from build123d import *

# Parameters (mm, degrees)
ENL_V_MAT_EXTRU_1_DEPTH      = 0.7
R_P_TITION_CIRCULAIRE1_COUNT = 4
ENL_V_MAT_EXTRU_2_REACH      = 75.418
ESQUISSE3_R                  = 1.25


with BuildPart() as part:
    # Esquisse1 → Révolution1 (revolve)
    with BuildSketch(Plane.XY, mode=Mode.PRIVATE) as r_volution1_sk:
        Polygon((0, 0), (0, 4), (0.45, 4), (2.7, 1.75), (43.2, 1.75), (43.2, 2), (72.8, 2), (73.2, 1.6), (73.2, 0), align=None)
    revolve(r_volution1_sk.sketch.rotate(Axis((0, 0, 0), (1, 0, 0)), 90), axis=Axis((0, 0, 0), (1, 0, 0)))

    # Esquisse2 → Enlèv. mat.-Extru.1 (cut, symmetric)
    with BuildSketch(Plane.XY):
        Polygon((0, 0), (0, 2.5), (0.5, 2), (2.5, 1.002836784), (2.5, 0), align=None)
    enl_v_mat_extru_1 = extrude(amount=ENL_V_MAT_EXTRU_1_DEPTH, both=True, mode=Mode.SUBTRACT)

    # Répétition circulaire1: Enlèv. mat.-Extru.1 ×4 about axis
    r_p_tition_circulaire1_axis = Axis((0, 0, 0), (1, 0, 0))
    for i in range(1, R_P_TITION_CIRCULAIRE1_COUNT):
        add(enl_v_mat_extru_1.rotate(r_p_tition_circulaire1_axis, i * 360 / R_P_TITION_CIRCULAIRE1_COUNT), mode=Mode.SUBTRACT)

    # Enlèv. mat.-Extru.2: up to this face of the body (flat: up to its plane)
    enl_v_mat_extru_2_end = Plane(part.part.faces().sort_by_distance((2.5, 0, 0))[0])
    # Esquisse3 → Enlèv. mat.-Extru.2 (cut, up to the picked face)
    with BuildSketch(Plane.ZY, mode=Mode.PRIVATE) as enl_v_mat_extru_2_sk1:
        with Locations(Location((0, 0, 0), (0, 0, 325.944202257))):
            Circle(ESQUISSE3_R)
    enl_v_mat_extru_2_tool1 = split(extrude(enl_v_mat_extru_2_sk1.sketch, amount=-ENL_V_MAT_EXTRU_2_REACH, mode=Mode.PRIVATE), bisect_by=enl_v_mat_extru_2_end, keep=Keep.BOTH, mode=Mode.PRIVATE)
    add(enl_v_mat_extru_2_tool1.solids().sort_by(Axis((0, 0, 0), (1, 0, 0)))[0], mode=Mode.SUBTRACT)


solid = part.part
Could you check a few things on this model? Use its own coordinates, in mm. A direction names the side the tool comes from. Coordinates: 2 decimals unless noted, no trailing zeros. Order: outer loops, then holes, each group sorted by start corner. A loop starts at its lowest first (then second) coordinate and runs counter-clockwise, first axis right, second up. Notation, with made-up numbers: (-35.75, -19.5) - (-15.75, -19.5) arc R21 cw to (-15.75, -6.5) - close; hole circle Ø1 at (28, 87). An arc over 180 degrees is marked (long way). Answer in a Markdown table with one row per item. Add a question column.
(1) If we mould it in two halves opening along Z, with no side actions, what happens to faces 1 (the face through (73.2, 0, 0)), 2 (the face through (2.5, 0, 0)), 3 (the face through (58, 2, 0))? For each: released by +Z, released by -Z, zero draft, split by the parting line, or undercut.
(2) If we section it at D-D, the plane x = 64.5: Please give me the cut outline in (y, z), then the cut area to 3 significant figures.
(3) Will these pins go through, and if not, where does the flat tip stop? pin 1 (1.6 mm diameter, centred on x = 2, y = 1.5, fed in from -Z); pin 2 (3 mm diameter, centred on x = 20.5, z = 0.5, fed in from +Y); pin 3 (2 mm diameter, centred on x = 16.5, y = 1.5, fed in from +Z); pin 4 (4.5 mm diameter, centred on y = 1, z = 0, fed in from -X).
(4) If we section it at B-B, the plane x = 23: Please give me the cut outline in (y, z), then the cut area to 3 significant figures.
(5) I need wall thicknesses on L1, parallel to Y at x = 0.95, z = 0; L2, parallel to Y at x = 1.9, z = 0; L3, parallel to Y at x = 50, z = -0.5. Which ranges of each line are inside material? Lowest first, please.
(6) If we section it at A-A, the plane z = 0: Please give me the cut outline in (x, y).
(7) On a 3-axis mill with a long thin cutter (end or side, diameter ignored), from which of +Z, -Z, +X, -X, +Y, -Y can I reach the whole of each face in a straight line? I mean faces 4 (the face through (0.228, 3.905, -0.867)), 5 (the face through (0.7, -0.7, 1.5)), 6 (the face through (23.23, 1.55, 0.81)). Say none if no direction works.
Results are:
| question | item | result |
|---|---|---|
| 1 | face 1 | zero draft |
| 1 | face 2 | undercut |
| 1 | face 3 | split by the parting line |
| 2 | outline | circle Ø4 at (0, 0) |
| 2 | area | 12.6 mm2 |
| 3 | pin 1 | stops at z = -2.96 |
| 3 | pin 2 | stops at y = 1.75 |
| 3 | pin 3 | stops at z = 1.68 |
| 3 | pin 4 | stops at x = 0 |
| 4 | outline | circle Ø3.5 at (0, 0) |
| 4 | area | 9.62 mm2 |
| 5 | L1 | y = -3.5 to -1.78, 1.78 to 3.5 |
| 5 | L2 | y = -2.55 to -1.3, 1.3 to 2.55 |
| 5 | L3 | y = -1.94 to 1.94 |
| 6 | outline | (0, -4) - (0.45, -4) - (2.7, -1.75) - (43.2, -1.75) - (43.2, -2) - (72.8, -2) - (73.2, -1.6) - (73.2, 1.6) - (72.8, 2) - (43.2, 2) - (43.2, 1.75) - (2.7, 1.75) - (0.45, 4) - (0, 4) - (0, 2.5) - (0.5, 2) - (2, 1.25) - (2.5, 1.25) - (2.5, -1.25) - (2, -1.25) - (0.5, -2) - (0, -2.5) - close |
| 7 | face 4 | +X, -X |
| 7 | face 5 | -X |
| 7 | face 6 | none |
